Answer from the drawing. Dimensions are ordinates in mm from the lowest x, y and z of the part. A direction names the side the tool comes from. Give positions to 0.01 mm unless a question says otherwise; leave off trailing zeros. Order: outer loops, then holes, each group sorted by start corner. A loop starts at its lowest first (then second) coordinate and runs counter-clockwise, first axis right, second up. Notation, with made-up numbers: M 55,-1.75 L 102,-1.75 A9 cw 102,3.25 Z; hole C 3.25,0.5 d11. An arc over 180 degrees is marked long. One line per item, written item: value.
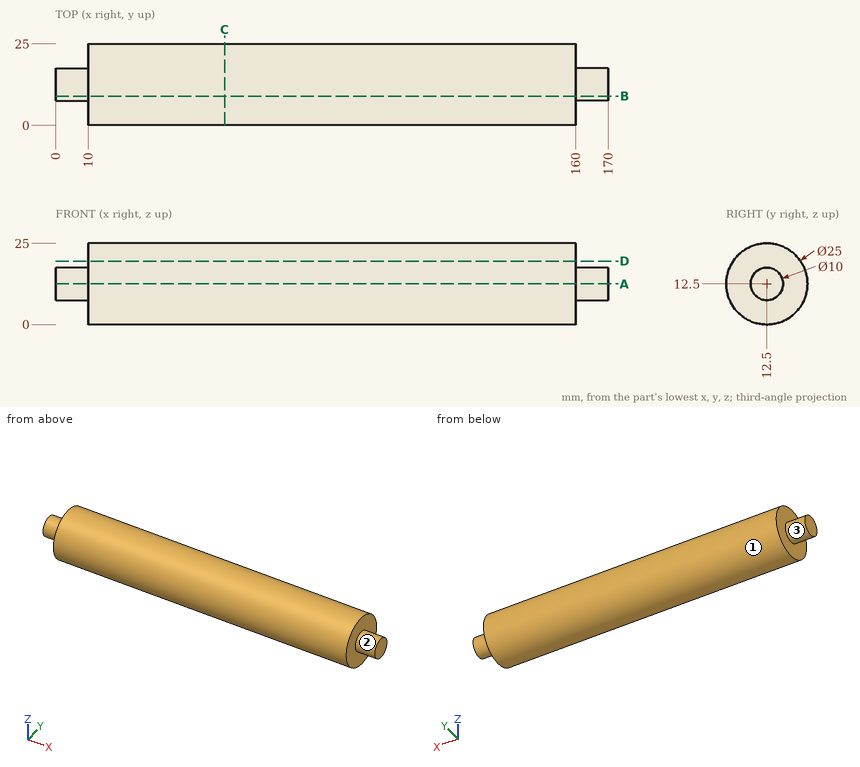
(1) Given P1, Ø12.5, axis at y = 13, z = 18, coming from the +X side; P2, Ø10, axis at x = 53.5, y = 3.5, coming from the -Z side; P3, Ø3, axis at x = 148.5, z = 6, coming from the -Y side; P4, Ø8, axis at y = 3, z = 5.5, coming from the -X side, each flat-ended and moving along its own axis, determine where each tip first touches the part or whether it passes through.
Findings:
P1: stops at x = 170
P2: stops at z = 0.66
P3: stops at y = 1.04
P4: stops at x = 10
(2) Section C-C, the plane x = 52 is taken. Give the vertices of the cut face in (y, z), then the cut area to 3 significant figures.
Findings:
outline: C 12.5,12.5 d25
area: 491 mm^2
(3) Section A-A, the plane z = 12.5 is taken. Give the vertices of the cut face in (x, y), then the cut area to 3 significant figures.
Findings:
outline: M 0,7.5 L 10,7.5 L 10,0 L 160,0 L 160,7.5 L 170,7.5 L 170,17.5 L 160,17.5 L 160,25 L 10,25 L 10,17.5 L 0,17.5 Z
area: 3,950 mm^2
(4) Find the intervals of material crossed by probe 1 along X at (y, z) = (19.75, 21); probe 2 along Z at (x, y) = (142, 11.75); probe 3 along Y at (x, z) = (58, 23.25), in increasing order. Write a range as from..to.
Findings:
probe 1: x = 10..160
probe 2: z = 0.02..24.98
probe 3: y = 6.12..18.88
(5) Which of the six approach directions +Z, -Z, +X, -X, +Y, -Y give full straight-line access (tool end or side, diameter ignored) to the marked faces 1, 2 and 3?
Findings:
face 1: +X, -X
face 2: +X
face 3: -X
(6) Section D-D, the plane z = 19.5 is taken. Give the vertices of the cut face in (x, y), then the cut area to 3 significant figures.
Findings:
outline: M 10,2.14 L 160,2.14 L 160,22.86 L 10,22.86 Z
area: 3,110 mm^2
(7) Section B-B, the plane y = 9 is taken. Give the vertices of the cut face in (x, z), then the cut area to 3 significant figures.
Findings:
outline: M 0,8.93 L 10,8.93 L 10,0.5 L 160,0.5 L 160,8.93 L 170,8.93 L 170,16.07 L 160,16.07 L 160,24.5 L 10,24.5 L 10,16.07 L 0,16.07 Z
area: 3,740 mm^2
